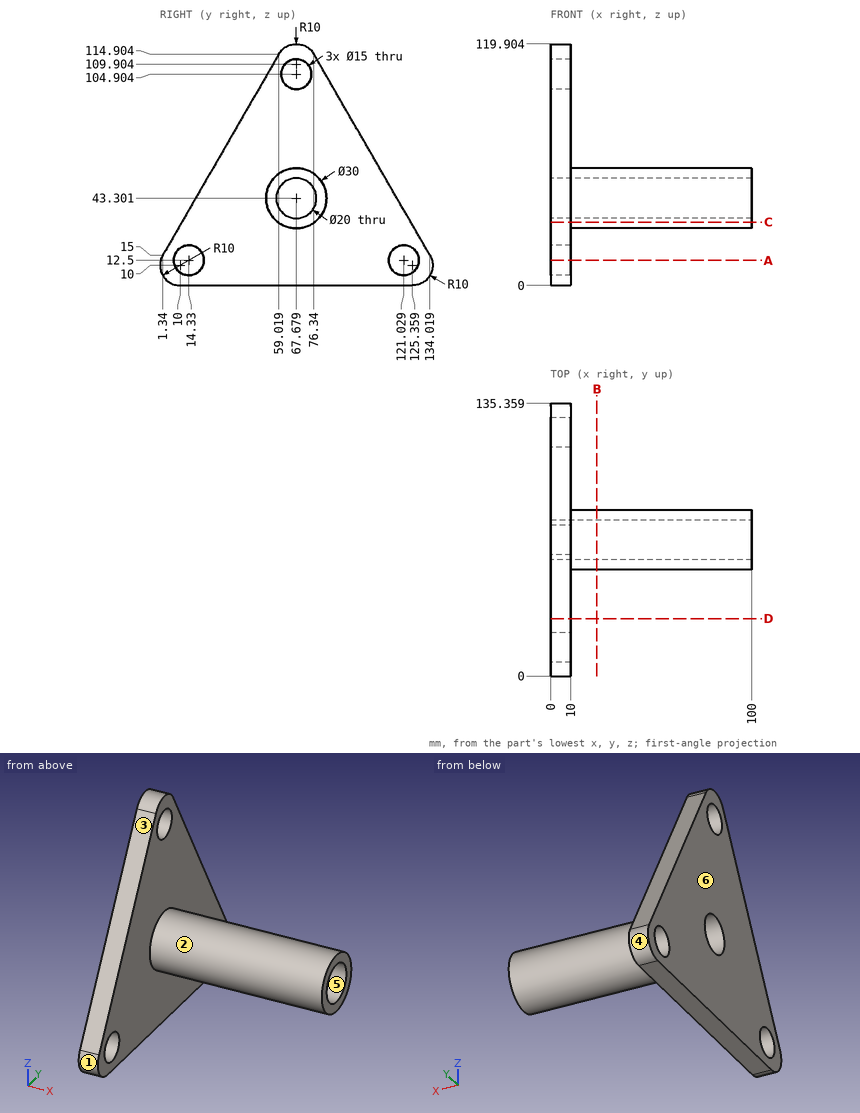
Here's the drawing with two shaded views (mm, measured from the low corner). I have some questions. A direction names the side the tool comes from. Coordinates: 2 decimals unless noted, no trailing zeros. Write each loop counter-clockwise with the first axis right and the second up, starting at its lowest first coordinate (ties: lowest second). Pieces come first, ordered by that corner, then holes. Notation, with made-up numbers: M -1.5,-17 L 57.5,-17 A22 ccw 57.5,9 Z; hole C 53.5,51 d6. An arc over 180 degrees is marked long. Use one line per item in the form item = value.
Q1. If we section it at B-B (x = 23): Write out the boundary of the cut face in (y, z).
Model answer:
outline = C 67.68,43.3 d30; hole C 67.68,43.3 d20
Q2. For the marked faces 1 and 2, which set-ups out of +Z, -Z, +X, -X, +Y, -Y let a thin tool reach every point of the face, with its end or its side?
Model answer:
face_1 = +X, -X, -Y
face_2 = +X
Q3. If we section it at D-D (y = 28.5): Write out the boundary of the cut face in (x, z).
Model answer:
outline = M 0,0 L 10,0 L 10,62.04 L 0,62.04 Z
Q4. I need wall thicknesses on line 1 along X through (y, z) = (102, 19.5); line 2 along Y through (x, z) = (12.5, 35) (1 decimal); line 3 along Z through (x, y) = (56, 65.5). Which ranges of each line are inside material? Lowest first, please. Write a range as from..to.
Model answer:
line_1 = 0..10
line_2 = 55.2..62.1, 73.3..80.2
line_3 = 28.46..33.54, 53.06..58.14
Q5. If we section it at C-C (z = 31.5): Write out the boundary of the cut face in (x, y).
Model answer:
outline = M 0,10.87 L 10,10.87 L 10,58.42 L 100,58.42 L 100,76.94 L 10,76.94 L 10,124.49 L 0,124.49 Z
Q6. If we section it at A-A (z = 12.5): Write out the boundary of the cut face in (x, y), then the cut area to 3 significant figures.
Model answer:
outline = M 0,0.32 L 10,0.32 L 10,6.83 L 0,6.83 Z; M 0,21.83 L 10,21.83 L 10,113.53 L 0,113.53 Z; M 0,128.53 L 10,128.53 L 10,135.04 L 0,135.04 Z
area = 1,050 mm^2
Q7. We'd pull the mould along Z, two halves only. Please class the marked faces 3, 4, 5 and 6: +Z half, -Z half, draft (parallel to the pull), parting line (faces both ways), or undercut.
Model answer:
face_3 = +Z half
face_4 = parting line
face_5 = undercut
face_6 = draft
Q8. For P1, Ø12, axis at y = 67.68, z = 104.9, coming from the +X side; P2, Ø3, axis at x = 23.5, y = 78, coming from the -Z side; P3, Ø8, axis at x = 35.5, y = 71.5, coming from the -Z side; P4, Ø2, axis at x = 73.5, y = 70, coming from the +Z side, each with a flat end and sliding along its axis, tell me the tip position at first contact or that it passes through.
Model answer:
P1 = through
P2 = 31.17
P3 = 28.3
P4 = 58.24
